The figure shows three views and two pictorial views of one solid part (mm, origin at its lowest corner). Answer the questions. Give positions to 0.01 mm unless a question says otherwise; leave off trailing zeros. Write each loop counter-clockwise with the first axis right and the second up, starting at its lowest first coordinate (ties: lowest second). Pieces come first, ordered by that corner, then holes. Notation, with made-up numbers: (80.25, 17) - (94.25, 17) arc R11 cw to (94.25, 36) - close; hole circle Ø3 at (52, 58.25). An arc over 180 degrees is marked (long way). Write each question's results on one line, items separated by ' | '. Start each with the question number.
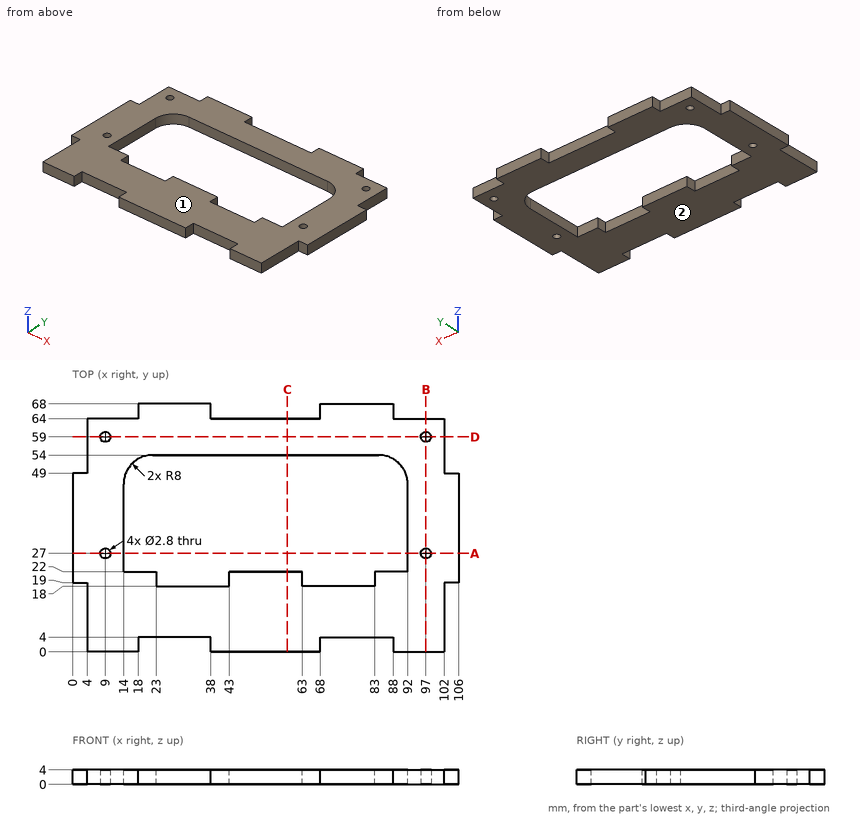
Q1. The mould has two halves that part along Z. Classify the marked faces 1 and 2: pulls with the +Z half, pulls with the -Z half, needs draft (parallel to the pull), parting line crosses it, or undercut.
Q2. A cutting plane is placed at D-D, the plane y = 59. Write down the section's boundary in (x, z).
Q3. Consider L1, parallel to Y at x = 9, z = 2.9; L2, parallel to X at y = 27, z = 2.5; L3, parallel to X at y = 59, z = 1. Determine where each line is inside the solid, lowest interval first.
Q4. Given pin 1 (2 mm diameter, centred on x = 49.5, z = 1.5, fed in from +Y); pin 2 (1.2 mm diameter, centred on x = 105, z = 2, fed in from +Y); pin 3 (2 mm diameter, centred on y = 1.5, z = 2, fed in from -X), each flat-ended and moving along its own axis, determine where each tip first touches the part or whether it passes through.
Q5. A cutting plane is placed at C-C, the plane x = 59. Write down the section's boundary in (y, z), and give its area (3 significant figures).
Q6. A cutting plane is placed at B-B, the plane x = 97. Write down the section's boundary in (y, z), and give its area (3 significant figures).
Q7. A cutting plane is placed at A-A, the plane y = 27. Write down the section's boundary in (x, z), and give its area (3 significant figures).
Result:
1) face 1: pulls with the +Z half | face 2: pulls with the -Z half
2) outline: (4, 0) - (7.6, 0) - (7.6, 4) - (4, 4) - close; (10.4, 0) - (95.6, 0) - (95.6, 4) - (10.4, 4) - close; (98.4, 0) - (102, 0) - (102, 4) - (98.4, 4) - close
3) L1: y = 0 to 25.6, 28.4 to 57.6, 60.4 to 64 | L2: x = 0 to 7.6, 10.4 to 14, 92 to 95.6, 98.4 to 106 | L3: x = 4 to 7.6, 10.4 to 95.6, 98.4 to 102
4) pin 1: stops at y = 64 | pin 2: stops at y = 49 | pin 3: stops at x = 4
5) outline: (0, 0) - (22, 0) - (22, 4) - (0, 4) - close; (54, 0) - (64, 0) - (64, 4) - (54, 4) - close | area: 128 mm2
6) outline: (0, 0) - (25.6, 0) - (25.6, 4) - (0, 4) - close; (28.4, 0) - (57.6, 0) - (57.6, 4) - (28.4, 4) - close; (60.4, 0) - (64, 0) - (64, 4) - (60.4, 4) - close | area: 234 mm2
7) outline: (0, 0) - (7.6, 0) - (7.6, 4) - (0, 4) - close; (10.4, 0) - (14, 0) - (14, 4) - (10.4, 4) - close; (92, 0) - (95.6, 0) - (95.6, 4) - (92, 4) - close; (98.4, 0) - (106, 0) - (106, 4) - (98.4, 4) - close | area: 89.6 mm2
